Could you check a few things on this model? Use its own coordinates, in mm. A direction names the side the tool comes from. Round coordinates to 2 decimals unless told otherwise and drop trailing zeros. Write each loop counter-clockwise with the first axis right and the second up, starting at its lowest first coordinate (ties: lowest second). Pieces come first, ordered by that corner, then holes. Notation, with made-up numbers: (-30.5, -16) - (21.5, -16) arc R19 cw to (21.5, 7) - close; hole circle Ø2 at (31.5, 38). An arc over 180 degrees is marked (long way). Put each result on its own line as item: value.
from build123d import *

# Parameters (mm, degrees)
F0_R     = 44.67
F0_R_2   = 42.07
F1_DEPTH = 6.75
F2_R     = 46.625
F2_R_2   = 42.16
F3_DEPTH = 2.73
F4_R     = 49.14
F4_R_2   = 46.25
F5_DEPTH = 9.5


with BuildPart() as f1:
    # F0 (on Front) → F1 (new body)
    with BuildSketch(Plane.XZ):
        Circle(F0_R)
        Circle(F0_R_2, mode=Mode.SUBTRACT)
    extrude(amount=F1_DEPTH)

    # F2 (on face) → F3 (join)
    with BuildSketch(Plane.XZ.offset(6.75)):
        Circle(F2_R)
        Circle(F2_R_2, mode=Mode.SUBTRACT)
    extrude(amount=F3_DEPTH)

    # F4 (on face) → F5 (join)
    with BuildSketch(Plane.XZ.offset(9.48)):
        Circle(F4_R)
        Circle(F4_R_2, mode=Mode.SUBTRACT)
    extrude(amount=F5_DEPTH)


solid = f1.part
(1) I'm going to push flat-ended pins straight in: pin 1 (6 mm diameter, centred on y = -10, z = -34.5, fed in from +X); pin 2 (3 mm diameter, centred on y = -6.5, z = -26.5, fed in from +X); pin 3 (10 mm diameter, centred on x = 13, y = -3, fed in from +Z). Where does each tip first touch, or does it pass through?
Values found:
pin 1: stops at x = 37.72
pin 2: stops at x = 39.34
pin 3: stops at z = 45.61
(2) Please list where these lines run through material, in increasing order: probe 1 along Z at (x, y) = (0, -7.5) (3 decimals); probe 2 along Z at (x, y) = (0, -15.5); probe 3 along X at (y, z) = (-1.5, -19). Write a range as from..to.
Values found:
probe 1: z = -46.625..-42.16, 42.16..46.625
probe 2: z = -49.14..-46.25, 46.25..49.14
probe 3: x = -40.43..-37.54, 37.54..40.43
(3) Imagine slicing it at A-A, the plane x = 0. List the corners of the cut face in (y, z) for me (3 decimals), then the cut area to 3 significant figures.
Values found:
outline: (-18.98, -49.14) - (-9.48, -49.14) - (-9.48, -46.625) - (-6.75, -46.625) - (-6.75, -44.67) - (0, -44.67) - (0, -42.07) - (-6.75, -42.07) - (-6.75, -42.16) - (-9.48, -42.16) - (-9.48, -46.25) - (-18.98, -46.25) - close; (-18.98, 46.25) - (-9.48, 46.25) - (-9.48, 42.16) - (-6.75, 42.16) - (-6.75, 42.07) - (0, 42.07) - (0, 44.67) - (-6.75, 44.67) - (-6.75, 46.625) - (-9.48, 46.625) - (-9.48, 49.14) - (-18.98, 49.14) - close
area: 114 mm^2
(4) Imagine slicing it at B-B, the plane z = 11. List the corners of the cut face in (x, y) for me.
Values found:
outline: (-47.89, -18.98) - (-44.92, -18.98) - (-44.92, -9.48) - (-40.7, -9.48) - (-40.7, -6.75) - (-40.61, -6.75) - (-40.61, 0) - (-43.29, 0) - (-43.29, -6.75) - (-45.31, -6.75) - (-45.31, -9.48) - (-47.89, -9.48) - close; (40.61, -6.75) - (40.7, -6.75) - (40.7, -9.48) - (44.92, -9.48) - (44.92, -18.98) - (47.89, -18.98) - (47.89, -9.48) - (45.31, -9.48) - (45.31, -6.75) - (43.29, -6.75) - (43.29, 0) - (40.61, 0) - close
(5) For faces 5 (the face through (40.127, -3.328, 12.637)), 6 (the face through (38, -6.75, -24)), 7 (the face through (24.86, -14.16, 39)), which set-ups out of +Z, -Z, +X, -X, +Y, -Y let a thin tool reach every point of the face, with its end or its side?
Values found:
face 5: +Y, -Y
face 6: +Y
face 7: -Y
(6) Imagine slicing it at D-D, the plane y = -1.5. List the corners of the cut face in (x, z) for me, then the cut area to 3 significant figures.
Values found:
outline: circle Ø89.34 at (0, 0); hole circle Ø84.14 at (0, 0)
area: 709 mm^2
(7) Imagine slicing it at C-C, the plane y = -8. List the corners of the cut face in (x, z) for me (3 decimals), then the cut area to 3 significant figures.
Values found:
outline: circle Ø93.25 at (0, 0); hole circle Ø84.32 at (0, 0)
area: 1,250 mm^2
(8) If we mould it in two halves opening along X, with no side actions, what happens to faces 1 (the face through (37.5, -9.48, -20.3)), 2 (the face through (24.01, -3.33, 37.67)), 3 (the face through (-33, -18.98, -33)), 4 (the face through (-33.46, -8.1, -25.65))? For each: pulls with the +X half, pulls with the -X half, needs draft (parallel to the pull), parting line crosses it, or undercut.
Values found:
face 1: undercut
face 2: parting line crosses it
face 3: needs draft
face 4: undercut
